Could you check a few things on this drawing? It's one solid part, dimensions in mm from its lowest x, y, z. A direction names the side the tool comes from. Coordinates: 2 decimals unless noted, no trailing zeros. Write each loop counter-clockwise with the first axis right and the second up, starting at its lowest first coordinate (ties: lowest second). Pieces come first, ordered by that corner, then holes.
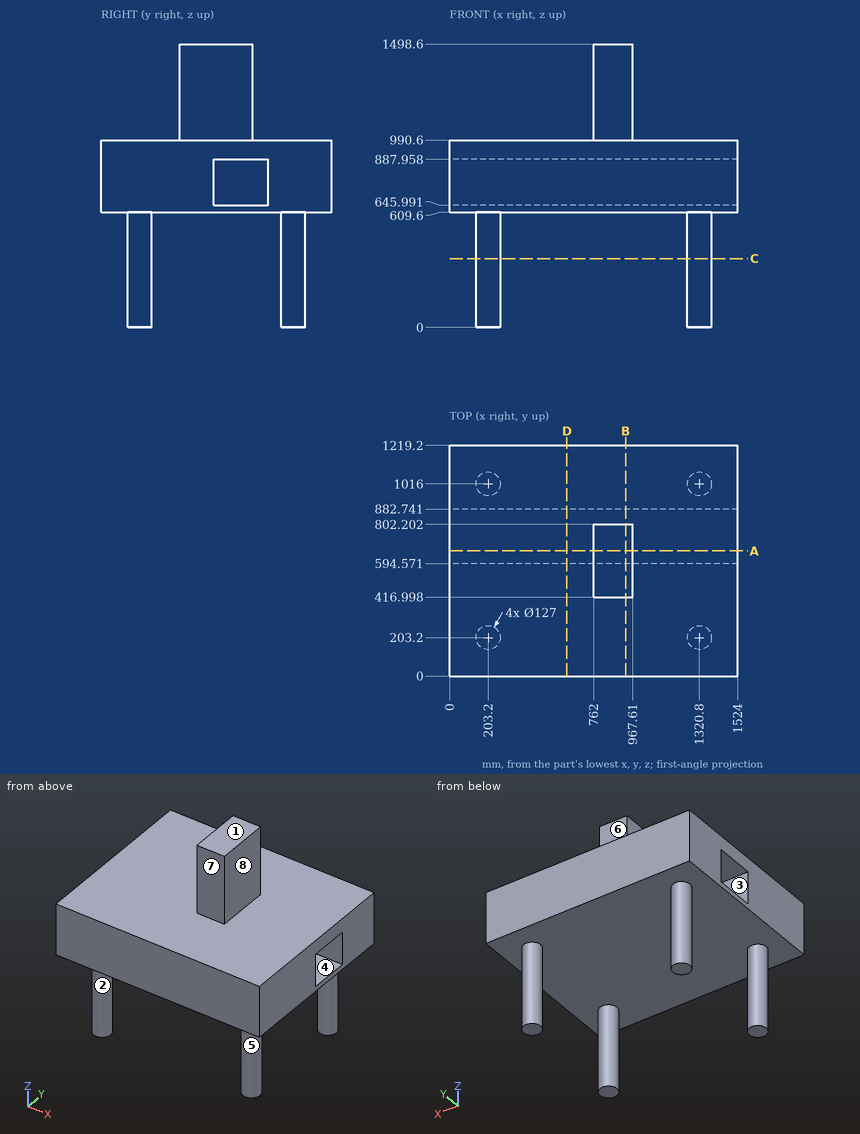
1) Imagine slicing it at B-B on x = 930. Please give me the cut outline in (y, z), then the cut area to 3 significant figures.
Values follow:
outline: (0, 609.6) - (1219.2, 609.6) - (1219.2, 990.6) - (802.2, 990.6) - (802.2, 1498.6) - (417, 1498.6) - (417, 990.6) - (0, 990.6) - close; hole (594.57, 645.99) - (882.74, 645.99) - (882.74, 887.96) - (594.57, 887.96) - close
area: 590,000 mm2
2) On a 3-axis mill with a long thin cutter (end or side, diameter ignored), from which of +Z, -Z, +X, -X, +Y, -Y can I reach the whole of each face in a straight line? I mean the marked faces 4, 5, 6, 7 and 8. Say none if no direction works.
Values follow:
face 4: +X, -X
face 5: -Z
face 6: +Z, +X, -X, +Y
face 7: +Z, +X, -X, -Y
face 8: +Z, +X, +Y, -Y
3) I need wall thicknesses on probe 1 along Y at (x, z) = (824, 873.5); probe 2 along Z at (x, y) = (514.5, 682); probe 3 along Z at (x, y) = (941.5, 330). Which ranges of each line are inside material? Lowest first, please.
Values follow:
probe 1: y = 0 to 594.57, 882.74 to 1219.2
probe 2: z = 609.6 to 645.99, 887.96 to 990.6
probe 3: z = 609.6 to 990.6
4) Imagine slicing it at C-C on z = 364. Please give me the cut outline in (x, y), then the cut area to 3 significant figures.
Values follow:
outline: circle Ø127 at (203.2, 203.2); circle Ø127 at (203.2, 1016); circle Ø127 at (1320.8, 203.2); circle Ø127 at (1320.8, 1016)
area: 50,700 mm2
5) Imagine slicing it at D-D on x = 619.5. Please give me the cut outline in (y, z).
Values follow:
outline: (0, 609.6) - (1219.2, 609.6) - (1219.2, 990.6) - (0, 990.6) - close; hole (594.57, 645.99) - (882.74, 645.99) - (882.74, 887.96) - (594.57, 887.96) - close
6) Will these pins go through, and if not, where does the flat tip stop? pin 1 (5 mm diameter, centred on y = 551, z = 1002, fed in from +X); pin 2 (12 mm diameter, centred on x = 759, y = 387, fed in from +Z); pin 3 (3 mm diameter, centred on x = 848.5, z = 1304.5, fed in from -Y).
Values follow:
pin 1: stops at x = 967.61
pin 2: stops at z = 990.6
pin 3: stops at y = 417
7) We'd pull the mould along Z, two halves only. Please class the marked faces 1, 2 and 3: pulls with the +Z half, pulls with the -Z half, needs draft (parallel to the pull), parting line crosses it, or undercut.
Values follow:
face 1: pulls with the +Z half
face 2: needs draft
face 3: undercut
8) Imagine slicing it at A-A on y = 662. Please give me the cut outline in (x, z).
Values follow:
outline: (0, 609.6) - (1524, 609.6) - (1524, 645.99) - (0, 645.99) - close; (0, 887.96) - (1524, 887.96) - (1524, 990.6) - (967.61, 990.6) - (967.61, 1498.6) - (762, 1498.6) - (762, 990.6) - (0, 990.6) - close
